from build123d import *

# Parameters (mm, degrees)
SKETCH_R             = 1.7
PAD_DEPTH            = 5
SKETCH_MIRRORED_2_R  = 1.7
PAD_MIRRORED_2_DEPTH = 5


with BuildPart() as part:
    # Sketch → Pad (new body)
    with BuildSketch(Plane.XY):
        with BuildLine():
            ThreePointArc((25, 0), (17.67767, 17.67767), (0, 25))
            Line((0, 25), (0, 0))
            Line((0, 0), (25, 0))
        make_face()
        with Locations((11.313708, 11.313708)):
            Circle(SKETCH_R, mode=Mode.SUBTRACT)
    pad = extrude(amount=PAD_DEPTH)

    # Sketch Mirrored 2 → Pad Mirrored 2 (add)
    with BuildSketch(Plane(origin=(0, 0, 0), x_dir=(-1, 0, 0), z_dir=(0, 0, -1))):
        with BuildLine():
            ThreePointArc((25, 0), (17.67767, 17.67767), (0, 25))
            Line((0, 25), (0, 0))
            Line((0, 0), (25, 0))
        make_face()
        with Locations((11.313708, 11.313708)):
            Circle(SKETCH_MIRRORED_2_R, mode=Mode.SUBTRACT)
    pad_mirrored_2 = extrude(amount=-PAD_MIRRORED_2_DEPTH)

    # Mirrored001: Pad, Pad Mirrored 2 across Sketch H_Axis
    add(pad.mirror(Plane.ZX))
    add(pad_mirrored_2.mirror(Plane.ZX))

    # Sketch001 → Groove (revolve, cut)
    with BuildSketch(Plane(origin=(2.5, 0, 0), x_dir=(1, 0, 0), z_dir=(0, -1, 0))):
        Polygon((0, 5), (4, 5), (4, 4), (8, 0), (0, 0), align=None)
    revolve(axis=Axis((2.5, 0, 0), (0, 0, 1)), mode=Mode.SUBTRACT)


solid = part.part
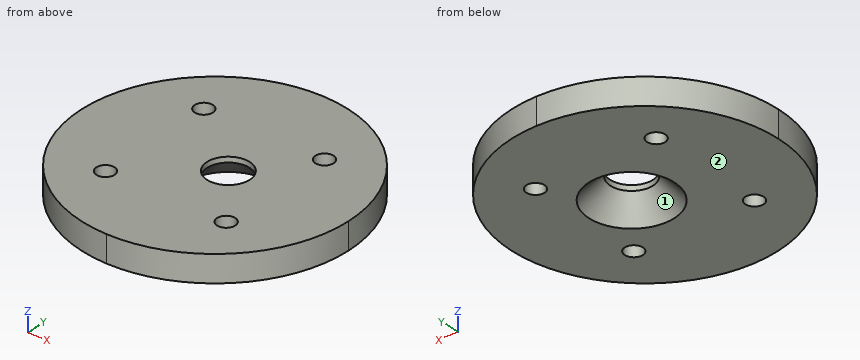
Design review of the part built by this model. Coordinates are the model's own, in mm. Face numbers are marked on the shaded views. Coordinates: 2 decimals unless noted, no trailing zeros. Order: outer loops, then holes, each group sorted by start corner. A loop starts at its lowest first (then second) coordinate and runs counter-clockwise, first axis right, second up. Notation, with made-up numbers: (-34, -35) -> (9, -35) arc R17 cw to (9, -15) -> close; hole circle Ø3 at (-8.75, 73.25). An arc over 180 degrees is marked (long way). Use one line per item in the form item = value. Start each with the question number.
(1) Add section D-D on x = -7. State the section outline as (y, z) points.
(2) For probe 1 along X at (y, z) = (-11, 0.95); probe 2 along X at (y, z) = (-5, 0.85); probe 3 along Y at (x, z) = (-10.5, 1.7), list the stretches that pass through material, from the lowest coordinate up.
(3) Add section C-C on z = 1.15. State the section outline as (x, y) points.
(4) Add section A-A on y = 10.5. State the section outline as (x, z) points.
(5) Add section B-B on x = 2.5. State the section outline as (y, z) points.
(6) The part is to be moulded in two halves that separate along Y. For the marked faces 1 and 2, say which applies: +Y half, -Y half, draft (parallel to the pull), parting line (faces both ways), or undercut.
(7) Insertion check: pin 1 (1 mm diameter, centred on y = 5, z = 3.5, fed in from +X); pin 2 (6 mm diameter, centred on x = -0.5, y = 1.5, fed in from -Z). Each pin has a flat end and moves straight along its axis. Give the tip position at first contact, or say it passes through.
Answer block:
q1.outline = (-24, 0) -> (24, 0) -> (24, 5) -> (-24, 5) -> close
q2.probe_1 = -22.45 to -12.98, -9.64 to 9.64, 12.98 to 22.45
q2.probe_2 = -24.49 to -2.61, 7.61 to 24.49
q2.probe_3 = -22.69 to -12.81, -9.82 to 9.82, 12.81 to 22.69
q3.outline = (-25, 0) arc R25 ccw to (0, -25) arc R25 ccw to (25, 0) arc R25 ccw to (0, 25) arc R25 ccw to start; hole circle Ø3.4 at (-11.31, -11.31); hole circle Ø3.4 at (-11.31, 11.31); hole circle Ø13.7 at (2.5, 0); hole circle Ø3.4 at (11.31, -11.31); hole circle Ø3.4 at (11.31, 11.31)
q4.outline = (-22.69, 0) -> (-12.81, 0) -> (-12.81, 5) -> (-22.69, 5) -> close; (-9.82, 0) -> (9.82, 0) -> (9.82, 5) -> (-9.82, 5) -> close; (12.81, 0) -> (22.69, 0) -> (22.69, 5) -> (12.81, 5) -> close
q5.outline = (-24.87, 0) -> (-8, 0) -> (-4, 4) -> (-4, 5) -> (-24.87, 5) -> close; (4, 4) -> (8, 0) -> (24.87, 0) -> (24.87, 5) -> (4, 5) -> close
q6.face_1 = undercut
q6.face_2 = draft
q7.pin_1 = 24.59
q7.pin_2 = 1.65
